Read the model definition and answer for the solid it produces. Units are mm, in the model's axes. Give positions to 0.01 mm unless a question says otherwise; leave off trailing zeros. Loops run counter-clockwise (first coordinate to the right, second up) from the corner with the lowest first, then second, coordinate; pieces in that order, holes last. Notation, with made-up numbers: (61, 60.25) - (84, 60.25) arc R12 ccw to (84, 73.25) - close; hole circle Ø9 at (9.25, 45). An arc over 180 degrees is marked (long way). Use a Markdown table: item, result. Add a question column.
Item 1: A cutting plane is placed at B-B (x = -33). Determine the outline of the cut face in (y, z).
Item 2: Each of these flat-tipped pins is pushed along its axis until it touches: P1, Ø3, axis at y = 3, z = 34, coming from the -X side; P2, Ø2.5, axis at x = -27.5, y = 3, coming from the -Z side; P3, Ø2.5, axis at x = -20.75, z = -35.94, coming from the +Y side; P4, Ø2.5, axis at x = 24.5, y = 3, coming from the -Z side. Where does it stop, or does it pass through?
Item 3: Consider probe 1 along X at (y, z) = (2.5, 26); probe 2 along X at (y, z) = (2.05, -23.5); probe 3 along Z at (x, y) = (22, 3.65). Determine where each line is inside the solid, lowest interval first. Write a range as [from, to].
Item 4: A cutting plane is placed at A-A (z = 0). Give the number of separate pieces and of enclosed holes in the cut face, plus the area to 3 significant figures.
Item 5: A cutting plane is placed at D-D (x = 26). Determine the outline of the cut face in (y, z), plus the area to 3 significant figures.
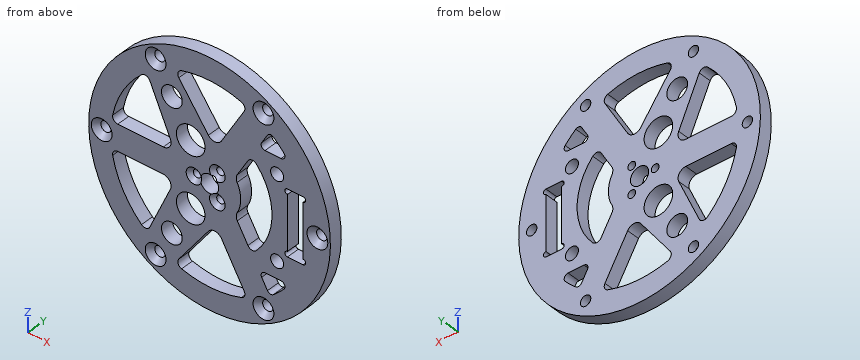
from build123d import *

# Parameters (mm, degrees)
SKETCH_1_R                = 46.5
SKETCH_1_R_2              = 2
SKETCH_1_R_3              = 3.5
SKETCH_1_R_4              = 2.5
SKETCH_1_R_5              = 4
SKETCH_1_R_6              = 1.5
SKETCH_1_W                = 6
SKETCH_1_H                = 25
EXTRUDE_1_DEPTH           = 5
HOLE_WIZARD_1_D           = 3
HOLE_WIZARD_1_CSINK_D     = 6
HOLE_WIZARD_1_CSINK_ANGLE = 90
HOLE_WIZARD_2_D           = 4
HOLE_WIZARD_2_CSINK_D     = 8
HOLE_WIZARD_2_CSINK_ANGLE = 90
SKETCH_4_R                = 1
CUT_EXTRUDE_1_DEPTH       = 66.9507392
SKETCH_5_R                = 5.5
CUT_EXTRUDE_2_DEPTH       = 66.9507392
FILLET_1_R                = 2
FILLET_2_R                = 3
FILLET_3_R                = 1.5


with BuildPart() as part:
    # 草图1 → 凸台-拉伸1 (new body)
    with BuildSketch(Plane(origin=(0, 0, 0), x_dir=(1, 0, 0), z_dir=(0, 1, 0))):
        with Locations(Location((0, 0, 0), (0, 0, 270))):
            Circle(SKETCH_1_R)
        with Locations(Location((-20.75, 35.940054257, 0), (0, 0, 270))):
            Circle(SKETCH_1_R_2, mode=Mode.SUBTRACT)
        with Locations(Location((20.75, 35.940054257, 0), (0, 0, 270))):
            Circle(SKETCH_1_R_2, mode=Mode.SUBTRACT)
        with Locations(Location((41.5, 0, 0), (0, 0, 270))):
            Circle(SKETCH_1_R_2, mode=Mode.SUBTRACT)
        with Locations(Location((20.75, -35.940054257, 0), (0, 0, 270))):
            Circle(SKETCH_1_R_2, mode=Mode.SUBTRACT)
        with Locations(Location((0, 0, 0), (0, 0, 270))):
            Circle(SKETCH_1_R_3, mode=Mode.SUBTRACT)
        with Locations(Location((-20.75, -35.940054257, 0), (0, 0, 270))):
            Circle(SKETCH_1_R_2, mode=Mode.SUBTRACT)
        with Locations(Location((-41.5, 0, 0), (0, 0, 270))):
            Circle(SKETCH_1_R_2, mode=Mode.SUBTRACT)
        with Locations(Location((26, 16, 0), (0, 0, 270))):
            Circle(SKETCH_1_R_4, mode=Mode.SUBTRACT)
        with Locations(Location((26, -16, 0), (0, 0, 270))):
            Circle(SKETCH_1_R_4, mode=Mode.SUBTRACT)
        with Locations(Location((-14.5, 25.11473671, 0), (0, 0, 270))):
            Circle(SKETCH_1_R_5, mode=Mode.SUBTRACT)
        with Locations(Location((-6, 0, 0), (0, 0, 270))):
            Circle(SKETCH_1_R_6, mode=Mode.SUBTRACT)
        with Locations(Location((3, 5.196152423, 0), (0, 0, 270))):
            Circle(SKETCH_1_R_6, mode=Mode.SUBTRACT)
        with Locations(Location((3, -5.196152423, 0), (0, 0, 270))):
            Circle(SKETCH_1_R_6, mode=Mode.SUBTRACT)
        with Locations(Location((-14.5, -25.11473671, 0), (0, 0, 270))):
            Circle(SKETCH_1_R_5, mode=Mode.SUBTRACT)
        with Locations((33, 0)):
            Rectangle(SKETCH_1_W, SKETCH_1_H, mode=Mode.SUBTRACT)
    extrude(amount=EXTRUDE_1_DEPTH)

    # 孔1 (through all)
    with Locations(Plane(origin=(0, 0, 0), x_dir=(-1, 0, 0), z_dir=(0, -1, 0))):
        with Locations((-3, 5.196152423), (6, 0), (-3, -5.196152423)):
            CounterSinkHole(HOLE_WIZARD_1_D / 2, HOLE_WIZARD_1_CSINK_D / 2, counter_sink_angle=HOLE_WIZARD_1_CSINK_ANGLE)

    # 孔2 (through all)
    with Locations(Plane(origin=(0, 0, 0), x_dir=(-1, 0, 0), z_dir=(0, -1, 0))):
        with Locations((-41.5, 0), (-20.75, 35.940054257), (20.75, 35.940054257), (41.5, 0), (20.75, -35.940054257), (-20.75, -35.940054257)):
            CounterSinkHole(HOLE_WIZARD_2_D / 2, HOLE_WIZARD_2_CSINK_D / 2, counter_sink_angle=HOLE_WIZARD_2_CSINK_ANGLE)

    # 草图4 → 切除-拉伸1 (cut, through all)
    with BuildSketch(Plane(origin=(0, 5, 0), x_dir=(1, 0, 0), z_dir=(0, 1, 0))):
        with Locations((30, 11.5)):
            Circle(SKETCH_4_R)
        with Locations((30, -11.5)):
            Circle(SKETCH_4_R)
        with Locations((36, -11.5)):
            Circle(SKETCH_4_R)
        with Locations((36, 11.5)):
            Circle(SKETCH_4_R)
    extrude(amount=-CUT_EXTRUDE_1_DEPTH, mode=Mode.SUBTRACT)

    # 草图5 → 切除-拉伸2 (cut, through all)
    with BuildSketch(Plane.XZ):
        with Locations(Location((-7.25, 12.557368355, 0), (0, 0, 270))):
            Circle(SKETCH_5_R)
        with Locations(Location((-7.25, -12.557368355, 0), (0, 0, 90))):
            Circle(SKETCH_5_R)
        with BuildLine():
            Line((-24.078608458, 29.397629407), (-13.184318354, 5))
            Line((-13.184318354, 5), (-37.669616404, 5))
            ThreePointArc((-37.669616404, 5), (-33.196715177, 18.49264993), (-24.078608458, 29.397629407))
        make_face()
        with BuildLine():
            Line((2.262032158, 13.917954626), (14.504681183, 35.122844756))
            ThreePointArc((14.504681183, 35.122844756), (0.583252966, 37.995523631), (-13.419789648, 35.551501316))
            Line((-13.419789648, 35.551501316), (2.262032158, 13.917954626))
        make_face()
        with BuildLine():
            Line((16.081480392, 17.8539411), (9.784483076, 6.947221814))
            ThreePointArc((9.784483076, 6.947221814), (12, 0), (9.784483076, -6.947221814))
            Line((9.784483076, -6.947221814), (16.081480392, -17.8539411))
            ThreePointArc((16.081480392, -17.8539411), (24.028675045, 0), (16.081480392, 17.8539411))
        make_face()
        with BuildLine():
            Line((23.164935221, 30.122844756), (18.763883749, 22.5))
            Line((18.763883749, 22.5), (30.622703996, 22.5))
            ThreePointArc((30.622703996, 22.5), (27.162556464, 26.574339622), (23.164935221, 30.122844756))
        make_face()
        with BuildLine():
            Line((18.763883749, -22.5), (30.622703996, -22.5))
            ThreePointArc((30.622703996, -22.5), (27.162556464, -26.574339622), (23.164935221, -30.122844756))
            Line((23.164935221, -30.122844756), (18.763883749, -22.5))
        make_face()
        with BuildLine():
            Line((2.262032158, -13.917954626), (14.504681183, -35.122844756))
            ThreePointArc((14.504681183, -35.122844756), (0.583252966, -37.995523631), (-13.419789648, -35.551501316))
            Line((-13.419789648, -35.551501316), (2.262032158, -13.917954626))
        make_face()
        with BuildLine():
            Line((-13.184318354, -5), (-37.669616404, -5))
            ThreePointArc((-37.669616404, -5), (-33.196715177, -18.49264993), (-24.078608458, -29.397629407))
            Line((-24.078608458, -29.397629407), (-13.184318354, -5))
        make_face()
    extrude(amount=-CUT_EXTRUDE_2_DEPTH, mode=Mode.SUBTRACT)

    # 圆角1
    fillet_1_edges = [part.edges().sort_by_distance(p)[0] for p in [
        (-13.419789648, 2.5, 35.551501316),
        (14.504681183, 2.5, 35.122844756),
        (16.081480392, 2.5, 17.8539411),
        (16.081480392, 2.5, -17.8539411),
        (-37.669616404, 2.5, 5),
        (-24.078608458, 2.5, 29.397629407),
        (-24.078608458, 2.5, -29.397629407),
        (-37.669616404, 2.5, -5),
        (14.504681183, 2.5, -35.122844756),
        (-13.419789648, 2.5, -35.551501316),
    ]]
    fillet(fillet_1_edges, radius=FILLET_1_R)

    # 圆角2
    fillet_2_edges = [part.edges().sort_by_distance(p)[0] for p in [
        (2.262032158, 2.5, 13.917954626),
        (9.784483076, 2.5, -6.947221814),
        (9.784483076, 2.5, 6.947221814),
        (-13.184318354, 2.5, 5),
        (-13.184318354, 2.5, -5),
        (2.262032158, 2.5, -13.917954626),
    ]]
    fillet(fillet_2_edges, radius=FILLET_2_R)

    # 圆角3
    fillet_3_edges = [part.edges().sort_by_distance(p)[0] for p in [
        (23.164935221, 2.5, 30.122844756),
        (30.622703996, 2.5, 22.5),
        (18.763883749, 2.5, 22.5),
        (23.164935221, 2.5, -30.122844756),
        (18.763883749, 2.5, -22.5),
        (30.622703996, 2.5, -22.5),
    ]]
    fillet(fillet_3_edges, radius=FILLET_3_R)


solid = part.part
Geometry says:
| question | item | result |
|---|---|---|
| 1 | outline | (0, -32.76) - (5, -32.76) - (5, -18.84) - (0, -18.84) - close; (0, -5) - (5, -5) - (5, 5) - (0, 5) - close; (0, 18.84) - (5, 18.84) - (5, 32.76) - (0, 32.76) - close |
| 2 | P1 | x = -33.26 |
| 2 | P2 | z = -38.38 |
| 2 | P3 | through |
| 2 | P4 | z = -40.27 |
| 3 | probe 1 | [-38.55, -27.71], [-22.56, -18.4], [-10.6, -6.5], [9.24, 20.78], [27.71, 38.55] |
| 3 | probe 2 | [-40.12, -29.86], [-21.45, -18.16], [-10.84, -4.68], [7.79, 19.95], [28.91, 40.12] |
| 3 | probe 3 | [-40.97, -37.5], [-34.38, -28.11], [-22.5, -9.66], [9.66, 22.5], [28.11, 34.38], [37.5, 40.97] |
| 4 | separate pieces | 7 |
| 4 | enclosed holes | 0 |
| 4 | area | 275 mm² |
| 5 | outline | (0, -38.55) - (5, -38.55) - (5, -27.71) - (0, -27.71) - close; (0, -22.5) - (5, -22.5) - (5, -18.5) - (0, -18.5) - close; (0, -13.5) - (5, -13.5) - (5, 13.5) - (0, 13.5) - close; (0, 18.5) - (5, 18.5) - (5, 22.5) - (0, 22.5) - close; (0, 27.71) - (5, 27.71) - (5, 38.55) - (0, 38.55) - close |
| 5 | area | 283 mm² |
